Autodesk Inventor part; units mm, degrees
ref_plane "YZ Plane" through (0, 0, 0) normal (1, 0, 0) x (0, 1, 0)
ref_plane "XZ Plane" through (0, 0, 0) normal (0, 1, 0) x (-1, 0, 0)
ref_plane "XY Plane" through (0, 0, 0) normal (0, 0, 1) x (1, 0, 0)
sketch "Sketch5" plane through (0, 0, 0) normal (0, 1, 0) x (-1, 0, 0)
  line L0 (0, 0) -> (29, 0)
  line L1 (29, 0) -> (29, 52.5)
  line L2 (29, 52.5) -> (0, 52.5)
  line L3 (0, 0) -> (0, 6)
  line L4 (0, 6) -> (19, 6)
  line L5 (19, 6) -> (19, 46.5)
  line L6 (19, 46.5) -> (0, 46.5)
  line L7 (0, 52.5) -> (0, 46.5)
  line L8 (0, 6) -> (0, 0)
  dimension "d96" = 29
  dimension "d97" = 52.5
  dimension "d98" = 6
  dimension "d99" = 19
  dimension "d101" = 40.5
extrude "Extrusion3" add sketch "Sketch5" along normal blind 32
sketch "Sketch6" plane through (-29, 0, 0) normal (-1, 0, 0) x (0, 0, 1)
  line L0 (26.25, 32) -> (41.25, 32)
  line L1 (41.25, 32) -> (41.25, 0)
  line L2 (41.25, 0) -> (11.25, 0)
  line L3 (11.25, 0) -> (11.25, 32)
  line L4 (11.25, 32) -> (26.25, 32)
  line L5 (0, 0) -> (52.5, 0)
  line L6 (0, 0) -> (0, 32)
  dimension "d106" = 15
  dimension "d107" = 32
  dimension "d108" = 30
  dimension "d109" = 32
  dimension "d110" = 0
  dimension "d111" = 11.25
extrude "Extrusion4" add sketch "Sketch6" along normal blind 21
hole "Hole8" at (-50, 15, 26.25) direction (1, 0, 0) diameter 19 depth 15 tip angle 118
properties part number "GARFO" material "Aluminium AW-7020"
Design review of the part built by this model. Coordinates are the model's own, in mm. A direction names the side the tool comes from. Round coordinates to 2 decimals unless told otherwise and drop trailing zeros. Loops run counter-clockwise (first coordinate to the right, second up) from the corner with the lowest first, then second, coordinate; pieces in that order, holes last. Notation, with made-up numbers: (43, 88) - (96, 88) arc R19 cw to (96, 110) - close; hole circle Ø2 at (13, 60). An arc over 180 degrees is marked (long way). One line per item, written item: value. Start each with the question number.
1) Insertion check: pin 1 Ø5 at (x, z) = (-15, 9.5) entering from -Y; pin 2 Ø10 at (x, z) = (-35, 9) entering from -Y; pin 3 Ø10.5 at (x, y) = (-36, 19) entering from +Z; pin 4 Ø12.5 at (y, z) = (9, 4.5) entering from -X. Each pin has a flat end and moves straight along its axis. Give the tip position at first contact, or say it passes through.
2) Consider section A-A on x = -44.5. Give the boundary of the cut face in (y, z).
3) For faces 1 (the flat face through (-19, 16, 26)), 2 (the flat face through (-29, 16, 6)), 3 (the flat face through (-39, 16, 41.25)), list the 3-axis set-ups (+Z, -Z, +X, -X, +Y, -Y) from which the entire face can be reached by the end or side of a thin tool; tool diameter is ignored.
4) Draft analysis for pull direction Z (two halves, no side actions). For faces 4 (the flat face through (-9, 16, 6)), 5 (the flat face through (-14, 16, 0)), 6 (the cylindrical face through (-42.4, 6.99, 31.36)), 7 (the flat face through (-30, 0, 27)), state which applies: +Z half, -Z half, draft (parallel to the pull), parting line (faces both ways), or undercut.
5) Consider section B-B on x = -7.5. Give the boundary of the cut face in (y, z).
6) To check wall thickness, follow L1, parallel to Y at x = -42.5, z = 26.25; L2, parallel to Z at x = -13, y = 12; L3, parallel to Z at x = -47, y = 15. State the ranges of each line that lie inside material, in increasing order. Write a range as from..to.
Reported:
1. pin 1: passes through
1. pin 2: stops at y = 0
1. pin 3: stops at z = 41.25
1. pin 4: stops at x = -29
2. outline: (0, 11.25) - (32, 11.25) - (32, 41.25) - (0, 41.25) - close; hole circle Ø19 at (15, 26.25)
3. face 1: +X, +Y, -Y
3. face 2: -Z, -X, +Y, -Y
3. face 3: +Z, -X, +Y, -Y
4. face 4: undercut
4. face 5: -Z half
4. face 6: undercut
4. face 7: draft
5. outline: (0, 0) - (32, 0) - (32, 6) - (0, 6) - close; (0, 46.5) - (32, 46.5) - (32, 52.5) - (0, 52.5) - close
6. L1: y = 0..5.5, 24.5..32
6. L2: z = 0..6, 46.5..52.5
6. L3: z = 11.25..16.75, 35.75..41.25
